```python
from build123d import *

# Parameters (mm, degrees)
SKETCH1_W               = 146
SKETCH1_H               = 20
BOSS_EXTRUDE1_DEPTH     = 2
SKETCH2_W               = 2
SKETCH2_H               = 20
BOSS_EXTRUDE2_DEPTH     = 18
CUT_EXTRUDE1_DEPTH      = 148.702403501
CUT_EXTRUDE1_DEPTH_BACK = 148.702403501
SKETCH3_R               = 2


with BuildPart() as part:
    # Sketch1 → Boss-Extrude1 (new body)
    with BuildSketch(Plane.XY):
        Rectangle(SKETCH1_W, SKETCH1_H)
    extrude(amount=BOSS_EXTRUDE1_DEPTH)

    # Sketch2 → Boss-Extrude2 (add)
    with BuildSketch(Plane.XY.offset(2)):
        with Locations((72, 0)):
            Rectangle(SKETCH2_W, SKETCH2_H)
        with Locations((-72, 0)):
            Rectangle(SKETCH2_W, SKETCH2_H)
    extrude(amount=BOSS_EXTRUDE2_DEPTH)

    # Sketch3 → Cut-Extrude1 (cut, two sides: drawn at the far end of the back side and taken through both)
    with BuildSketch(Plane.ZY.offset(73).offset(-CUT_EXTRUDE1_DEPTH_BACK)):
        with Locations((10, 0)):
            Circle(SKETCH3_R)
    extrude(amount=CUT_EXTRUDE1_DEPTH + CUT_EXTRUDE1_DEPTH_BACK, mode=Mode.SUBTRACT)


solid = part.part
```
CAD build for the part. Positions are in the model's coordinates, mm. A direction names the side the tool comes from. Coordinates: 2 decimals unless noted, no trailing zeros. Order: outer loops, then holes, each group sorted by start corner. A loop starts at its lowest first (then second) coordinate and runs counter-clockwise, first axis right, second up. Notation, with made-up numbers: M 89.25,51 L 95.25,51 A21 ccw 95.25,90 Z; hole C 77,46.5 d2. An arc over 180 degrees is marked long. Write each question's results on one line, items separated by ' | '. Start each with the question number.
Q1. Pull direction X, two halves, no side cores. Call faces 1 (the flat face through (-73, -2.4, 9.9)), 2 (the flat face through (-1, 0, 2)), 3 (the flat face through (-1, 0, 0)): +X half, -X half, draft (parallel to the pull), parting line (faces both ways), or undercut.
Q2. Cut at B-B (y = 0). List the corners of the cut face in (x, z).
Q3. Cut at C-C (x = -2). List the corners of the cut face in (y, z).
Q4. Cut at A-A (z = 13.25). List the corners of the cut face in (x, y), then the cut area to 3 significant figures.
Q5. Which spindle directions (+Z, -Z, +X, -X, +Y, -Y) get a long thin tool onto all of the face, cutting with end or side? Do faces 4 (the flat face through (71, 0, 13)), 5 (the flat face through (0, -10, 1)). Say none if no direction does.
Q6. Drill centre lines: probe 1 along Z at (x, y) = (-71.75, 0); probe 2 along X at (y, z) = (4, 12.25); probe 3 along Y at (x, z) = (72, 10). Where is each one in solid material? Low to high. Write a range as from..to.
Q7. Flat gauge pins, fed straight in: P1, Ø3, axis at x = 2.5, y = -5, coming from the -Z side; P2, Ø3, axis at y = 0, z = 10, coming from the +X side; P3, Ø12, axis at x = 43, y = 7.5, coming from the +Z side. Where does each tip first touch, or does it go through?
Found:
1) face 1: -X half | face 2: undercut | face 3: draft
2) outline: M -73,0 L 73,0 L 73,8 L 71,8 L 71,2 L -71,2 L -71,8 L -73,8 Z; M -73,12 L -71,12 L -71,20 L -73,20 Z; M 71,12 L 73,12 L 73,20 L 71,20 Z
3) outline: M -10,0 L 10,0 L 10,2 L -10,2 Z
4) outline: M -73,-10 L -71,-10 L -71,10 L -73,10 Z; M 71,-10 L 73,-10 L 73,10 L 71,10 Z | area: 80.0 mm²
5) face 4: +Z, +Y, -Y | face 5: +Z, -Z, +X, -X, -Y
6) probe 1: 0..8, 12..20 | probe 2: -73..-71, 71..73 | probe 3: -10..-2, 2..10
7) P1: z = 0 | P2: through | P3: z = 2
